Build history of the part. All positions in model axes, mm. A direction names the side the tool comes from. Give positions to 0.01 mm unless a question says otherwise; leave off trailing zeros. Write each loop counter-clockwise with the first axis right and the second up, starting at its lowest first coordinate (ties: lowest second). Pieces come first, ordered by that corner, then holes. Notation, with made-up numbers: (32.5, 88.5) -> (49.5, 88.5) arc R19 ccw to (49.5, 108.5) -> close; hole circle Ø5 at (21, 60). An arc over 180 degrees is marked (long way). Write item = value, one per line. Start each with the question number.
Q1. Saw through at C-C, the plane z = 0.7. List the corners of the cut face in (x, y).
Q2. Drop a flat-ended pin along its axis: P1, Ø1.5, axis at y = 6, z = -1.5, coming from the -X side. Give the stop position or say it passes through.
Q3. Saw through at D-D, the plane x = 0.8. List the corners of the cut face in (y, z), then the cut area to 3 significant figures.
Q4. Saw through at A-A, the plane x = 0. List the corners of the cut face in (y, z).
Q5. Tool access for faces 1 (the face through (0.65, 16.23, -1.01)), 2 (the face through (0, 7, -2.2)), 3 (the face through (-2.3, 11, -1)): list every direction of +Z, -Z, +X, -X, +Y, -Y with a clear straight run to the whole face (end or side of a thin tool).
Q6. Saw through at B-B, the plane y = 3.75. List the corners of the cut face in (x, z).
Q7. Wall check: line 1 (Z direction, x = -0.1, y = 12); line 2 (Y direction, x = 0.1, z = 0.95); line 3 (Y direction, x = 0.4, z = 2). Give the ranges that are in metal, low to high.
from build123d import *

# Parameters (mm, degrees)
ESBO_O2_R                = 2
RESSALTO_EXTRUS_O1_DEPTH = 15
ESBO_O3_R                = 1.2
RESSALTO_EXTRUS_O2_DEPTH = 2.5
ESBO_O4_R                = 0.35
RESSALTO_EXTRUS_O3_DEPTH = 1.4
ESBO_O5_R                = 2.3
ESBO_O5_R_2              = 2
RESSALTO_EXTRUS_O4_DEPTH = 8
ESBO_O6_R                = 2.3
ESBO_O6_W                = 4.6
ESBO_O6_H                = 3
RESSALTO_EXTRUS_O6_DEPTH = 8


with BuildPart() as part:
    # Esboço2 → Ressalto-extrusão1 (new body)
    with BuildSketch(Plane(origin=(0, 0, 0), x_dir=(1, 0, 0), z_dir=(0, 1, 0))):
        Circle(ESBO_O2_R)
    extrude(amount=RESSALTO_EXTRUS_O1_DEPTH)

    # Esboço3 → Ressalto-extrusão2 (add)
    with BuildSketch(Plane(origin=(0, 15, 0), x_dir=(1, 0, 0), z_dir=(0, 1, 0))):
        Circle(ESBO_O3_R)
    extrude(amount=RESSALTO_EXTRUS_O2_DEPTH)

    # Esboço4 → Ressalto-extrusão3 (add)
    with BuildSketch(Plane(origin=(0, 17.5, 0), x_dir=(1, 0, 0), z_dir=(0, 1, 0))):
        Circle(ESBO_O4_R)
    extrude(amount=RESSALTO_EXTRUS_O3_DEPTH)

    # Esboço5 → Ressalto-extrusão4 (add)
    with BuildSketch(Plane(origin=(0, 15, 0), x_dir=(1, 0, 0), z_dir=(0, 1, 0))):
        Circle(ESBO_O5_R)
        Circle(ESBO_O5_R_2, mode=Mode.SUBTRACT)
    extrude(amount=-RESSALTO_EXTRUS_O4_DEPTH)

    # Esboço6 → Ressalto-extrusão6 (add)
    with BuildSketch(Plane(origin=(0, 15, 0), x_dir=(1, 0, 0), z_dir=(0, 1, 0))):
        Circle(ESBO_O6_R)
        with Locations((0, 1.5)):
            Rectangle(ESBO_O6_W, ESBO_O6_H)
    extrude(amount=-RESSALTO_EXTRUS_O6_DEPTH)


solid = part.part
Report:
q1.outline = (-2.19, 7) -> (-1.87, 7) -> (-1.87, 0) -> (1.87, 0) -> (1.87, 7) -> (2.19, 7) -> (2.19, 15) -> (0.97, 15) -> (0.97, 17.5) -> (-0.97, 17.5) -> (-0.97, 15) -> (-2.19, 15) -> close
q2.P1 = -1.85
q3.outline = (0, -1.83) -> (7, -1.83) -> (7, -3) -> (15, -3) -> (15, -0.89) -> (17.5, -0.89) -> (17.5, 0.89) -> (15, 0.89) -> (15, 2.16) -> (7, 2.16) -> (7, 1.83) -> (0, 1.83) -> close
q3.area = 71.4 mm2
q4.outline = (0, -2) -> (7, -2) -> (7, -3) -> (15, -3) -> (15, -1.2) -> (17.5, -1.2) -> (17.5, -0.35) -> (18.9, -0.35) -> (18.9, 0.35) -> (17.5, 0.35) -> (17.5, 1.2) -> (15, 1.2) -> (15, 2.3) -> (7, 2.3) -> (7, 2) -> (0, 2) -> close
q5.face_1 = +Y
q5.face_2 = -Y
q5.face_3 = +Z, -Z, -X, +Y, -Y
q6.outline = circle Ø4 at (0, 0)
q7.line_1 = -3 to 2.3
q7.line_2 = 0 to 17.5
q7.line_3 = 7 to 15
